Work out the finished part from the listing and answer in its coordinate system (mm). Give positions to 0.01 mm unless a question says otherwise; leave off trailing zeros. Write each loop counter-clockwise with the first axis right and the second up, starting at its lowest first coordinate (ties: lowest second). Pieces come first, ordered by that corner, then holes. Notation, with made-up numbers: (57, -34.75) - (116, -34.75) arc R16 ccw to (116, -14.75) - close; hole circle Ø4 at (-32, 38). An arc over 180 degrees is marked (long way). Write item = value, one per line.
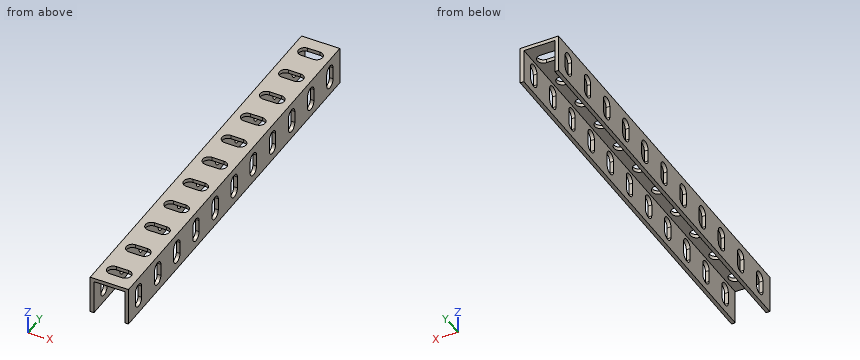
from build123d import *

# Parameters (mm, degrees)
SKETCH1_W           = 13.54
SKETCH1_H           = 140
BOSS_EXTRUDE1_DEPTH = 1.3
SKETCH5_W           = 13.54
SKETCH5_H           = 140
BOSS_EXTRUDE2_DEPTH = 1.3


with BuildPart() as part:
    # Sketch1 → Boss-Extrude1 (new body)
    with BuildSketch(Plane.XY):
        with Locations((0, -63.33)):
            Rectangle(SKETCH1_W, SKETCH1_H)
        with BuildLine():
            Line((-2.15, 2.11), (2.15, 2.11))
            ThreePointArc((2.15, 2.11), (4.26, 0), (2.15, -2.11))
            Line((2.15, -2.11), (-2.15, -2.11))
            ThreePointArc((-2.15, -2.11), (-4.26, 0), (-2.15, 2.11))
        make_face(mode=Mode.SUBTRACT)
        with BuildLine():
            Line((-2.15, -10.57), (2.15, -10.57))
            ThreePointArc((2.15, -10.57), (4.26, -12.68), (2.15, -14.79))
            Line((2.15, -14.79), (-2.15, -14.79))
            ThreePointArc((-2.15, -14.79), (-4.26, -12.68), (-2.15, -10.57))
        make_face(mode=Mode.SUBTRACT)
        with BuildLine():
            Line((-2.15, -23.25), (2.15, -23.25))
            ThreePointArc((2.15, -23.25), (4.26, -25.36), (2.15, -27.47))
            Line((2.15, -27.47), (-2.15, -27.47))
            ThreePointArc((-2.15, -27.47), (-4.26, -25.36), (-2.15, -23.25))
        make_face(mode=Mode.SUBTRACT)
        with BuildLine():
            Line((-2.15, -35.93), (2.15, -35.93))
            ThreePointArc((2.15, -35.93), (4.26, -38.04), (2.15, -40.15))
            Line((2.15, -40.15), (-2.15, -40.15))
            ThreePointArc((-2.15, -40.15), (-4.26, -38.04), (-2.15, -35.93))
        make_face(mode=Mode.SUBTRACT)
        with BuildLine():
            Line((-2.15, -48.61), (2.15, -48.61))
            ThreePointArc((2.15, -48.61), (4.26, -50.72), (2.15, -52.83))
            Line((2.15, -52.83), (-2.15, -52.83))
            ThreePointArc((-2.15, -52.83), (-4.26, -50.72), (-2.15, -48.61))
        make_face(mode=Mode.SUBTRACT)
        with BuildLine():
            Line((-2.15, -61.29), (2.15, -61.29))
            ThreePointArc((2.15, -61.29), (4.26, -63.4), (2.15, -65.51))
            Line((2.15, -65.51), (-2.15, -65.51))
            ThreePointArc((-2.15, -65.51), (-4.26, -63.4), (-2.15, -61.29))
        make_face(mode=Mode.SUBTRACT)
        with BuildLine():
            Line((-2.15, -73.97), (2.15, -73.97))
            ThreePointArc((2.15, -73.97), (4.26, -76.08), (2.15, -78.19))
            Line((2.15, -78.19), (-2.15, -78.19))
            ThreePointArc((-2.15, -78.19), (-4.26, -76.08), (-2.15, -73.97))
        make_face(mode=Mode.SUBTRACT)
        with BuildLine():
            Line((-2.15, -86.65), (2.15, -86.65))
            ThreePointArc((2.15, -86.65), (4.26, -88.76), (2.15, -90.87))
            Line((2.15, -90.87), (-2.15, -90.87))
            ThreePointArc((-2.15, -90.87), (-4.26, -88.76), (-2.15, -86.65))
        make_face(mode=Mode.SUBTRACT)
        with BuildLine():
            Line((-2.15, -99.33), (2.15, -99.33))
            ThreePointArc((2.15, -99.33), (4.26, -101.44), (2.15, -103.55))
            Line((2.15, -103.55), (-2.15, -103.55))
            ThreePointArc((-2.15, -103.55), (-4.26, -101.44), (-2.15, -99.33))
        make_face(mode=Mode.SUBTRACT)
        with BuildLine():
            Line((-2.15, -112.01), (2.15, -112.01))
            ThreePointArc((2.15, -112.01), (4.26, -114.12), (2.15, -116.23))
            Line((2.15, -116.23), (-2.15, -116.23))
            ThreePointArc((-2.15, -116.23), (-4.26, -114.12), (-2.15, -112.01))
        make_face(mode=Mode.SUBTRACT)
        with BuildLine():
            Line((-2.15, -124.69), (2.15, -124.69))
            ThreePointArc((2.15, -124.69), (4.26, -126.8), (2.15, -128.91))
            Line((2.15, -128.91), (-2.15, -128.91))
            ThreePointArc((-2.15, -128.91), (-4.26, -126.8), (-2.15, -124.69))
        make_face(mode=Mode.SUBTRACT)
    extrude(amount=-BOSS_EXTRUDE1_DEPTH)

    # Sketch5 → Boss-Extrude2 (add)
    with BuildSketch(Plane(origin=(6.77, 0, 0), x_dir=(0, 0, -1), z_dir=(1, 0, 0))):
        with Locations((6.77, -63.33)):
            Rectangle(SKETCH5_W, SKETCH5_H)
        with BuildLine():
            Line((4.62, 2.25), (8.92, 2.25))
            ThreePointArc((8.92, 2.25), (11.03, 0.14), (8.92, -1.97))
            Line((8.92, -1.97), (4.62, -1.97))
            ThreePointArc((4.62, -1.97), (2.51, 0.14), (4.62, 2.25))
        make_face(mode=Mode.SUBTRACT)
        with BuildLine():
            Line((4.62, -10.43), (8.92, -10.43))
            ThreePointArc((8.92, -10.43), (11.03, -12.54), (8.92, -14.65))
            Line((8.92, -14.65), (4.62, -14.65))
            ThreePointArc((4.62, -14.65), (2.51, -12.54), (4.62, -10.43))
        make_face(mode=Mode.SUBTRACT)
        with BuildLine():
            Line((4.62, -23.11), (8.92, -23.11))
            ThreePointArc((8.92, -23.11), (11.03, -25.22), (8.92, -27.33))
            Line((8.92, -27.33), (4.62, -27.33))
            ThreePointArc((4.62, -27.33), (2.51, -25.22), (4.62, -23.11))
        make_face(mode=Mode.SUBTRACT)
        with BuildLine():
            Line((4.62, -35.79), (8.92, -35.79))
            ThreePointArc((8.92, -35.79), (11.03, -37.9), (8.92, -40.01))
            Line((8.92, -40.01), (4.62, -40.01))
            ThreePointArc((4.62, -40.01), (2.51, -37.9), (4.62, -35.79))
        make_face(mode=Mode.SUBTRACT)
        with BuildLine():
            Line((4.62, -48.47), (8.92, -48.47))
            ThreePointArc((8.92, -48.47), (11.03, -50.58), (8.92, -52.69))
            Line((8.92, -52.69), (4.62, -52.69))
            ThreePointArc((4.62, -52.69), (2.51, -50.58), (4.62, -48.47))
        make_face(mode=Mode.SUBTRACT)
        with BuildLine():
            Line((4.62, -61.15), (8.92, -61.15))
            ThreePointArc((8.92, -61.15), (11.03, -63.26), (8.92, -65.37))
            Line((8.92, -65.37), (4.62, -65.37))
            ThreePointArc((4.62, -65.37), (2.51, -63.26), (4.62, -61.15))
        make_face(mode=Mode.SUBTRACT)
        with BuildLine():
            Line((4.62, -73.83), (8.92, -73.83))
            ThreePointArc((8.92, -73.83), (11.03, -75.94), (8.92, -78.05))
            Line((8.92, -78.05), (4.62, -78.05))
            ThreePointArc((4.62, -78.05), (2.51, -75.94), (4.62, -73.83))
        make_face(mode=Mode.SUBTRACT)
        with BuildLine():
            Line((4.62, -86.51), (8.92, -86.51))
            ThreePointArc((8.92, -86.51), (11.03, -88.62), (8.92, -90.73))
            Line((8.92, -90.73), (4.62, -90.73))
            ThreePointArc((4.62, -90.73), (2.51, -88.62), (4.62, -86.51))
        make_face(mode=Mode.SUBTRACT)
        with BuildLine():
            Line((4.62, -99.19), (8.92, -99.19))
            ThreePointArc((8.92, -99.19), (11.03, -101.3), (8.92, -103.41))
            Line((8.92, -103.41), (4.62, -103.41))
            ThreePointArc((4.62, -103.41), (2.51, -101.3), (4.62, -99.19))
        make_face(mode=Mode.SUBTRACT)
        with BuildLine():
            Line((4.62, -111.87), (8.92, -111.87))
            ThreePointArc((8.92, -111.87), (11.03, -113.98), (8.92, -116.09))
            Line((8.92, -116.09), (4.62, -116.09))
            ThreePointArc((4.62, -116.09), (2.51, -113.98), (4.62, -111.87))
        make_face(mode=Mode.SUBTRACT)
        with BuildLine():
            Line((4.62, -124.55), (8.92, -124.55))
            ThreePointArc((8.92, -124.55), (11.03, -126.66), (8.92, -128.77))
            Line((8.92, -128.77), (4.62, -128.77))
            ThreePointArc((4.62, -128.77), (2.51, -126.66), (4.62, -124.55))
        make_face(mode=Mode.SUBTRACT)
    boss_extrude2 = extrude(amount=-BOSS_EXTRUDE2_DEPTH)

    # Mirror1: Boss-Extrude2 across plane
    add(boss_extrude2.mirror(Plane(origin=(0, 0, 0), x_dir=(0, 0, 1), z_dir=(1, 0, 0))))


solid = part.part
1. Given pin 1 (3 mm diameter, centred on x = 1.5, y = -27, fed in from -Z); pin 2 (8 mm diameter, centred on x = -2, y = -26.5, fed in from -Z), each flat-ended and moving along its own axis, determine where each tip first touches the part or whether it passes through.
Solution:
pin_1 = -1.3
pin_2 = -13.54
2. Find section A-A, the plane y = -114.12. Give the vertices of the cut face in (x, z), then the cut area to 3 significant figures.
Solution:
outline = (-6.77, -13.54) - (-5.47, -13.54) - (-5.47, -11.03) - (-6.77, -11.03) - close; (-6.77, -2.51) - (-5.47, -2.51) - (-5.47, -1.3) - (-4.26, -1.3) - (-4.26, 0) - (-6.77, 0) - close; (4.26, -1.3) - (5.47, -1.3) - (5.47, -2.51) - (6.77, -2.51) - (6.77, 0) - (4.26, 0) - close; (5.47, -13.54) - (6.77, -13.54) - (6.77, -11.03) - (5.47, -11.03) - close
area = 16.2 mm^2
3. Find section B-B, the plane x = -0.5. Give the number of separate pieces and of enclosed holes in the cut face, then the cut area to 3 significant figures.
Solution:
separate_pieces = 12
enclosed_holes = 0
area = 122 mm^2
4. Straight lines are drawn through the part: line 1 (X direction, y = -74.5, z = -11.5); line 2 (Z direction, x = 3.5, y = -68); line 3 (Z direction, x = -6, y = -100). For each, find the intervals that lie inside material, in ascending order.
Solution:
line_1 = -6.77 to -5.47, 5.47 to 6.77
line_2 = -1.3 to 0
line_3 = -13.54 to -10.58, -2.96 to 0
5. Find section C-C, the plane y = -46. Give the vertices of the cut face in (x, z).
Solution:
outline = (-6.77, -13.54) - (-5.47, -13.54) - (-5.47, -1.3) - (5.47, -1.3) - (5.47, -13.54) - (6.77, -13.54) - (6.77, 0) - (-6.77, 0) - close
